```python
from build123d import *

# Parameters (mm, degrees)
SKETCH1_W           = 70.41
SKETCH1_H           = 58.37
SKETCH1_W_2         = 66.41
SKETCH1_H_2         = 54.37
BOSS_EXTRUDE1_DEPTH = 4
SKETCH2_W           = 70.41
SKETCH2_H           = 58.37
SKETCH2_W_2         = 35.9
SKETCH2_H_2         = 29.9
BOSS_EXTRUDE2_DEPTH = 1.5
FILLET1_R           = 0.56
BOSS_EXTRUDE3_DEPTH = 1


with BuildPart() as part:
    # Sketch1 → Boss-Extrude1 (new body)
    with BuildSketch(Plane(origin=(0, 0, 0), x_dir=(1, 0, 0), z_dir=(0, 1, 0))):
        Rectangle(SKETCH1_W, SKETCH1_H)
        Rectangle(SKETCH1_W_2, SKETCH1_H_2, mode=Mode.SUBTRACT)
    extrude(amount=BOSS_EXTRUDE1_DEPTH)

    # Sketch2 → Boss-Extrude2 (add)
    with BuildSketch(Plane(origin=(0, 4, 0), x_dir=(1, 0, 0), z_dir=(0, 1, 0))):
        Rectangle(SKETCH2_W, SKETCH2_H)
        Rectangle(SKETCH2_W_2, SKETCH2_H_2, mode=Mode.SUBTRACT)
    extrude(amount=BOSS_EXTRUDE2_DEPTH)

    # Fillet1
    fillet1_edges = [part.edges().sort_by_distance(p)[0] for p in [
        (17.95, 4.75, -14.95),
        (-17.95, 4.75, -14.95),
        (-17.95, 4.75, 14.95),
        (17.95, 4.75, 14.95),
    ]]
    fillet(fillet1_edges, radius=FILLET1_R)

    # Sketch3 → Boss-Extrude3 (add)
    with BuildSketch(Plane.XZ.offset(-4)):
        with BuildLine():
            Line((18.95, -14.45), (18.95, 14.45))
            ThreePointArc((18.95, 14.45), (18.510660172, 15.510660172), (17.45, 15.95))
            Line((17.45, 15.95), (-17.45, 15.95))
            ThreePointArc((-17.45, 15.95), (-18.510660172, 15.510660172), (-18.95, 14.45))
            Line((-18.95, 14.45), (-18.95, -14.45))
            ThreePointArc((-18.95, -14.45), (-18.510660172, -15.510660172), (-17.45, -15.95))
            Line((-17.45, -15.95), (17.45, -15.95))
            ThreePointArc((17.45, -15.95), (18.510660172, -15.510660172), (18.95, -14.45))
        make_face()
        with BuildLine():
            Line((17.45, -14.95), (-17.45, -14.95))
            ThreePointArc((-17.45, -14.95), (-17.803553391, -14.803553391), (-17.95, -14.45))
            Line((-17.95, -14.45), (-17.95, 14.45))
            ThreePointArc((-17.95, 14.45), (-17.803553391, 14.803553391), (-17.45, 14.95))
            Line((-17.45, 14.95), (17.45, 14.95))
            ThreePointArc((17.45, 14.95), (17.803553391, 14.803553391), (17.95, 14.45))
            Line((17.95, 14.45), (17.95, -14.45))
            ThreePointArc((17.95, -14.45), (17.803553391, -14.803553391), (17.45, -14.95))
        make_face(mode=Mode.SUBTRACT)
    extrude(amount=BOSS_EXTRUDE3_DEPTH)


solid = part.part
```
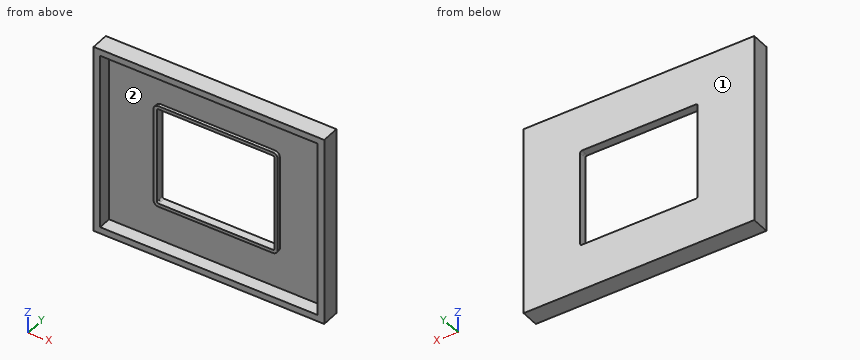
Work out the finished part from the listing and answer in its coordinate system (mm). Face numbers are marked on the shaded views. Round coordinates to 2 decimals unless told otherwise and drop trailing zeros. Order: outer loops, then holes, each group sorted by start corner. A loop starts at its lowest first (then second) coordinate and runs counter-clockwise, first axis right, second up.
Q1. A cutting plane is placed at D-D, the plane x = -25.5. Determine the outline of the cut face in (y, z) (3 decimals), then the cut area to 3 significant figures.
Solution:
outline: (0, -29.185) - (5.5, -29.185) - (5.5, 29.185) - (0, 29.185) - (0, 27.185) - (4, 27.185) - (4, -27.185) - (0, -27.185) - close
area: 104 mm2
Q2. The mould has two halves that part along X. Classify the marked faces 1 and 2: pulls with the +X half, pulls with the -X half, needs draft (parallel to the pull), parting line crosses it, or undercut.
Solution:
face 1: needs draft
face 2: undercut
Q3. A cutting plane is placed at C-C, the plane y = 1.7. Determine the outline of the cut face in (x, z) (3 decimals), then the cut area to 3 significant figures.
Solution:
outline: (-35.205, -29.185) - (35.205, -29.185) - (35.205, 29.185) - (-35.205, 29.185) - close; hole (-33.205, -27.185) - (33.205, -27.185) - (33.205, 27.185) - (-33.205, 27.185) - close
area: 499 mm2
Q4. Given pin 1 Ø0.6 at (x, z) = (18, -14.5) entering from -Y, flat-ended and moving along its own axis, determine where the tip first touches the part or whether it passes through.
Solution:
pin 1: stops at y = 3
Q5. A cutting plane is placed at A-A, the plane x = 12. Determine the outline of the cut face in (y, z) (3 decimals).
Solution:
outline: (0, -29.185) - (5.5, -29.185) - (5.5, -14.95) - (3, -14.95) - (3, -15.95) - (4, -15.95) - (4, -27.185) - (0, -27.185) - close; (0, 27.185) - (4, 27.185) - (4, 15.95) - (3, 15.95) - (3, 14.95) - (5.5, 14.95) - (5.5, 29.185) - (0, 29.185) - close
Q6. A cutting plane is placed at B-B, the plane z = -2.5. Determine the outline of the cut face in (x, y) (3 decimals), then the cut area to 3 significant figures.
Solution:
outline: (-35.205, 0) - (-33.205, 0) - (-33.205, 4) - (-18.95, 4) - (-18.95, 3) - (-17.95, 3) - (-17.95, 5.5) - (-35.205, 5.5) - close; (17.95, 3) - (18.95, 3) - (18.95, 4) - (33.205, 4) - (33.205, 0) - (35.205, 0) - (35.205, 5.5) - (17.95, 5.5) - close
area: 69.8 mm2
Q7. Find the intervals of material crossed by line 1 along X through (y, z) = (3.15, -4.5) (3 decimals); line 2 along X through (y, z) = (2.7, 0) (3 decimals); line 3 along Z through (x, y) = (-13, 4.75) (3 decimals), in increasing order.
Solution:
line 1: x = -35.205 to -33.205, -18.95 to -17.95, 17.95 to 18.95, 33.205 to 35.205
line 2: x = -35.205 to -33.205, 33.205 to 35.205
line 3: z = -29.185 to -14.95, 14.95 to 29.185
